The model under review builds one solid part; all positions refer to its coordinate system, in mm. A direction names the side the tool comes from. Round coordinates to 2 decimals unless told otherwise and drop trailing zeros. Loops run counter-clockwise (first coordinate to the right, second up) from the corner with the lowest first, then second, coordinate; pieces in that order, holes last. Notation, with made-up numbers: M -35.75,78 L -8.75,78 A18 ccw -8.75,107 Z; hole C 2,38.5 d2. An arc over 180 degrees is marked long. Return JSON: item names as keys, results as strings. Group by question number.
Q1. Consider section B-B (x = 0). State the section outline as (y, z) points (3 decimals), and give its area (3 significant figures).
Q2. For faces 1 (the face through (-0.22, 9.06, 19.64)), 2 (the face through (24.783, 7.304, 0.366)), list the 3-axis set-ups (+Z, -Z, +X, -X, +Y, -Y) from which the entire face can be reached by the end or side of a thin tool; tool diameter is ignored.
Q3. Clearance check with flat-ended pins moving along their axes: pin 1 Ø5 at (x, y) = (-18, 9) entering from -Z; pin 2 Ø1 at (x, y) = (0.5, 7.5) entering from +Z; pin 3 Ø1 at (x, y) = (-12, 5.5) entering from +Z. State where each tip first meets the part, or that it passes through.
Q4. Consider section A-A (z = 20). State the section outline as (x, y) points (3 decimals), and give its area (3 significant figures).
Q5. To check wall thickness, follow line 1 along Y through (x, z) = (0, 18); line 2 along X through (y, z) = (5.75, -7); line 3 along X through (y, z) = (13.5, 3.5). State the ranges of each line that lie inside material, in increasing order.
Q6. Consider section D-D (y = 3.5). State the section outline as (x, z) points.
Q7. Consider section C-C (z = -0.5). State the section outline as (x, y) points (3 decimals).
Q8. Draft analysis for pull direction Y (two halves, no side actions). For faces 3 (the face through (0, 14.816, 0)), 4 (the face through (0, 7, 13.97)), 5 (the face through (-0.4, 4, 24.2)), state which applies: pulls with the +Y half, pulls with the -Y half, needs draft (parallel to the pull), parting line crosses it, or undercut.
from build123d import *

# Parameters (mm, degrees)
ESQUISSE1_W             = 46.99
ESQUISSE1_H             = 46.99
BOSS_EXTRU_1_DEPTH      = 14.81582
BOSS_EXTRU_1_DRAFT      = -10
ESQUISSE4_R             = 1.666875
ENL_V_MAT_EXTRU_1_DEPTH = 12.7


with BuildPart() as part:
    # Esquisse1 → Boss.-Extru.1 (with draft: the straight prism first)
    with BuildSketch(Plane(origin=(0, 0, 0), x_dir=(1, 0, 0), z_dir=(0, 1, 0))):
        Rectangle(ESQUISSE1_W, ESQUISSE1_H)
    extrude(amount=BOSS_EXTRU_1_DEPTH)
    # Boss.-Extru.1: the draft: its side faces are tilted about the plane it starts from
    boss_extru_1_sides = [part.faces().sort_by_distance(p)[0] for p in [
        (0, 7.40791, 23.495),
        (23.495, 7.40791, 0),
        (0, 7.40791, -23.495),
        (-23.495, 7.40791, 0),
    ]]
    draft(boss_extru_1_sides, Plane(origin=(0, 0, 0), x_dir=(1, 0, 0), z_dir=(0, 1, 0)), BOSS_EXTRU_1_DRAFT)

    # Esquisse4 → Enlèv. mat.-Extru.1 (cut)
    with BuildSketch(Plane.XY.offset(26.67)):
        with Locations((0, 7.40791)):
            Circle(ESQUISSE4_R)
    extrude(amount=-ENL_V_MAT_EXTRU_1_DEPTH, mode=Mode.SUBTRACT)


solid = part.part
Values:
{
 "1": {"outline": "M 0,-23.495 L 14.816,-26.107 L 14.816,26.107 L 9.075,25.095 L 9.075,13.97 L 5.741,13.97 L 5.741,24.507 L 0,23.495 Z", "area": "699 mm2"},
 "2": {"face 1": "+Z", "face 2": "+Z, -Z, +X, -Y"},
 "3": {"pin 1": "stops at z = -25.52", "pin 2": "stops at z = 13.97", "pin 3": "stops at z = 24.55"},
 "4": {"outline": "M -26.107,14.816 L -23.495,0 L 23.495,0 L 26.107,14.816 Z; hole C 0,7.408 d3.334", "area": "726 mm2"},
 "5": {"line 1": "y = 0 to 5.74, 9.07 to 14.82", "line 2": "x = -24.51 to 24.51", "line 3": "x = -25.88 to 25.88"},
 "6": {"outline": "M -24.11,-24.11 L 24.11,-24.11 L 24.11,24.11 L -24.11,24.11 Z"},
 "7": {"outline": "M -26.107,14.816 L -23.495,0 L 23.495,0 L 26.107,14.816 Z"},
 "8": {"face 3": "pulls with the +Y half", "face 4": "undercut", "face 5": "pulls with the -Y half"}
}
